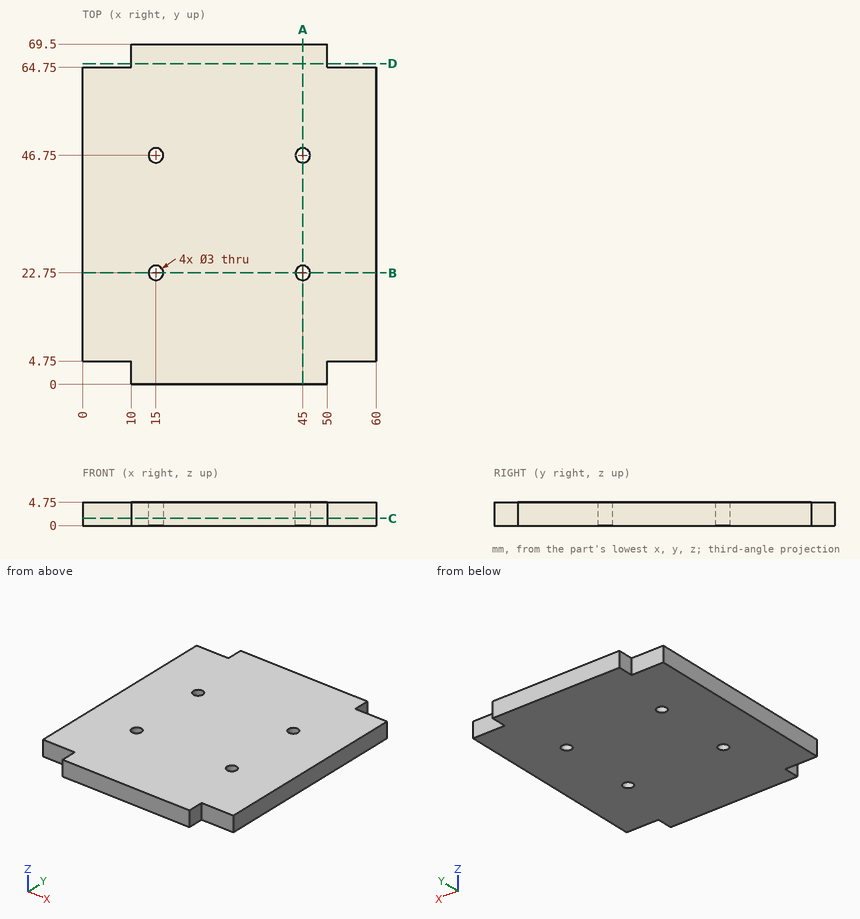
For this review, use the dimensioned drawing (mm, ordinates from the lowest corner) and the shaded views. Round coordinates to 2 decimals unless told otherwise and drop trailing zeros. Order: outer loops, then holes, each group sorted by start corner. A loop starts at its lowest first (then second) coordinate and runs counter-clockwise, first axis right, second up. Notation, with made-up numbers: M 88.25,89 L 131.25,89 A28 cw 131.25,124 Z; hole C 34.5,-39.5 d9. An arc over 180 degrees is marked long. Write each question's results on one line, items separated by ' | '. Start each with the question number.
1. Add section D-D (y = 65.5). State the section outline as (x, z) points, then the cut area to 3 significant figures.
2. Add section A-A (x = 45). State the section outline as (y, z) points.
3. To check wall thickness, follow L1, parallel to Y at x = 15, z = 3.1; L2, parallel to Y at x = 16, z = 4.4; L3, parallel to Y at x = 4, z = 2.95. State the ranges of each line that lie inside material, in increasing order. Write a range as [from, to].
4. Add section B-B (y = 22.75). State the section outline as (x, z) points, then the cut area to 4 significant figures.
5. Clearance check with flat-ended pins moving along their axes: pin 1 Ø1.4 at (x, z) = (5, 1.5) entering from +Y; pin 2 Ø2.5 at (y, z) = (1.5, 1.5) entering from -X; pin 3 Ø6 at (x, y) = (38.5, 17.5) entering from -Z; pin 4 Ø2.5 at (x, y) = (45, 46.75) entering from -Z. State where each tip first meets the part, or that it passes through.
6. Add section C-C (z = 1.45). State the section outline as (x, y) points.
Output values:
1) outline: M 10,0 L 50,0 L 50,4.75 L 10,4.75 Z | area: 190 mm^2
2) outline: M 0,0 L 21.25,0 L 21.25,4.75 L 0,4.75 Z; M 24.25,0 L 45.25,0 L 45.25,4.75 L 24.25,4.75 Z; M 48.25,0 L 69.5,0 L 69.5,4.75 L 48.25,4.75 Z
3) L1: [0, 21.25], [24.25, 45.25], [48.25, 69.5] | L2: [0, 21.63], [23.87, 45.63], [47.87, 69.5] | L3: [4.75, 64.75]
4) outline: M 0,0 L 13.5,0 L 13.5,4.75 L 0,4.75 Z; M 16.5,0 L 43.5,0 L 43.5,4.75 L 16.5,4.75 Z; M 46.5,0 L 60,0 L 60,4.75 L 46.5,4.75 Z | area: 256.5 mm^2
5) pin 1: y = 64.75 | pin 2: x = 10 | pin 3: z = 0 | pin 4: through
6) outline: M 0,4.75 L 10,4.75 L 10,0 L 50,0 L 50,4.75 L 60,4.75 L 60,64.75 L 50,64.75 L 50,69.5 L 10,69.5 L 10,64.75 L 0,64.75 Z; hole C 15,22.75 d3; hole C 15,46.75 d3; hole C 45,22.75 d3; hole C 45,46.75 d3
